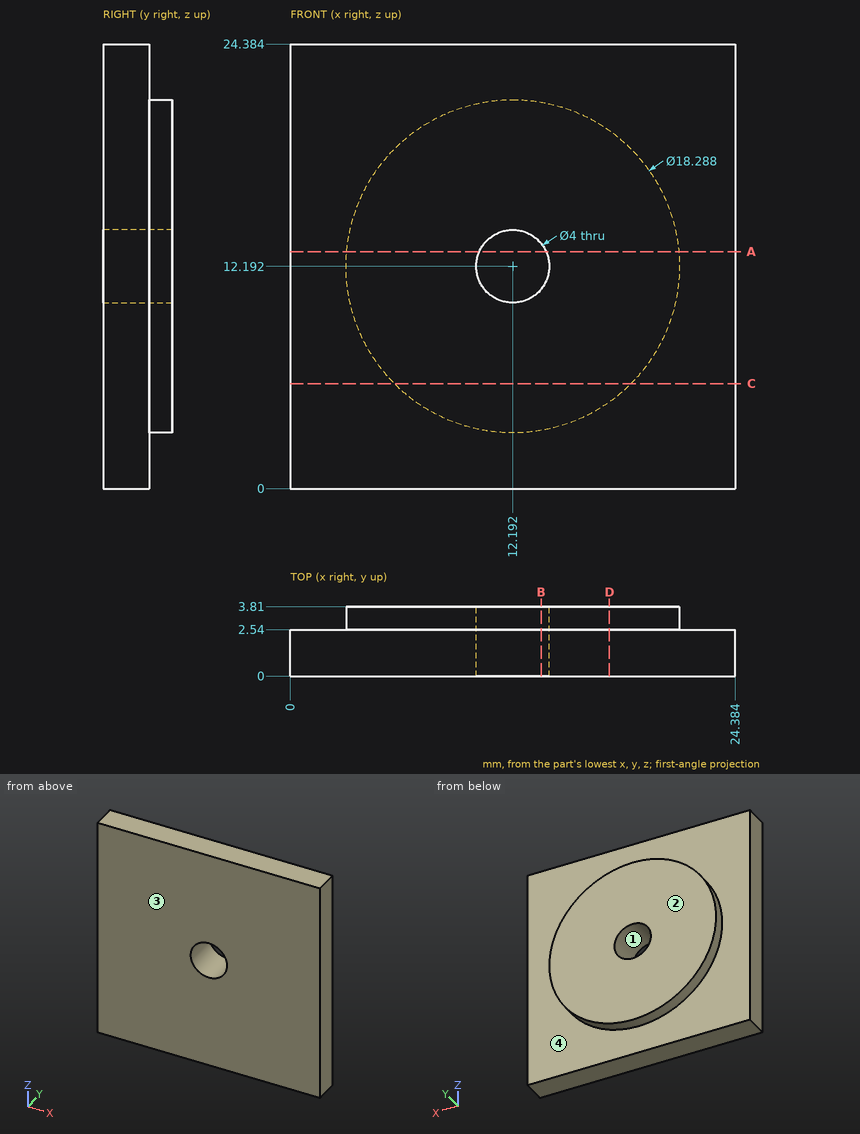
Could you check a few things on this drawing? It's one solid part, dimensions in mm from its lowest x, y, z. A direction names the side the tool comes from. Give positions to 0.01 mm unless a question says otherwise; leave off trailing zeros. Write each loop counter-clockwise with the first axis right and the second up, starting at its lowest first coordinate (ties: lowest second). Pieces come first, ordered by that corner, then holes. Notation, with made-up numbers: (85, 2) -> (130, 2) arc R35 cw to (130, 35) -> close; hole circle Ø4 at (39, 60). An arc over 180 degrees is marked (long way). Answer as a JSON object with one key per item and string values.
Q1. Suppose I cut it at D-D on x = 17.5. Write out the boundary of the cut face in (y, z), then the cut area to 3 significant figures.
Taken from the geometry:
{"outline": "(0, 0) -> (2.54, 0) -> (2.54, 4.75) -> (3.81, 4.75) -> (3.81, 19.64) -> (2.54, 19.64) -> (2.54, 24.38) -> (0, 24.38) -> close", "area": "80.8 mm²"}
Q2. Please list where these lines run through material, in increasing order: L1, parallel to Y at x = 19.25, z = 4; L2, parallel to X at y = 0.4, z = 13; L3, parallel to X at y = 3.6, z = 12.
Taken from the geometry:
{"L1": "y = 0 to 2.54", "L2": "x = 0 to 10.36, 14.02 to 24.38", "L3": "x = 3.05 to 10.2, 14.18 to 21.33"}
Q3. We'd pull the mould along X, two halves only. Please class the marked faces 1 and 2: released by +X, released by -X, zero draft, split by the parting line, or undercut.
Taken from the geometry:
{"face 1": "undercut", "face 2": "zero draft"}
Q4. Which directions (+Z, -Z, +X, -X, +Y, -Y) give clear straight access to the entire face, cutting with the end or side of a thin tool? Please do the marked faces 3 and 4.
Taken from the geometry:
{"face 3": "+Z, -Z, +X, -X, -Y", "face 4": "+Y"}
Q5. Suppose I cut it at C-C on z = 5.75. Write out the boundary of the cut face in (x, y).
Taken from the geometry:
{"outline": "(0, 0) -> (24.38, 0) -> (24.38, 2.54) -> (18.68, 2.54) -> (18.68, 3.81) -> (5.7, 3.81) -> (5.7, 2.54) -> (0, 2.54) -> close"}
Q6. Suppose I cut it at A-A on z = 13. Write out the boundary of the cut face in (x, y), then the cut area to 3 significant figures.
Taken from the geometry:
{"outline": "(0, 0) -> (10.36, 0) -> (10.36, 3.81) -> (3.08, 3.81) -> (3.08, 2.54) -> (0, 2.54) -> close; (14.02, 0) -> (24.38, 0) -> (24.38, 2.54) -> (21.3, 2.54) -> (21.3, 3.81) -> (14.02, 3.81) -> close", "area": "71.1 mm²"}
Q7. Suppose I cut it at B-B on x = 13.75. Write out the boundary of the cut face in (y, z).
Taken from the geometry:
{"outline": "(0, 0) -> (2.54, 0) -> (2.54, 3.18) -> (3.81, 3.18) -> (3.81, 10.94) -> (0, 10.94) -> close; (0, 13.45) -> (3.81, 13.45) -> (3.81, 21.2) -> (2.54, 21.2) -> (2.54, 24.38) -> (0, 24.38) -> close"}
Q8. Will these pins go through, and if not, where does the flat tip stop? pin 1 Ø5 at (x, z) = (6, 17.5) entering from -Y; pin 2 Ø2.5 at (x, z) = (12.192, 12.192) entering from +Y.
Taken from the geometry:
{"pin 1": "stops at y = 0", "pin 2": "passes through"}
